Read the model definition and answer for the solid it produces. Units are mm, in the model's axes. A direction names the side the tool comes from. Round coordinates to 2 decimals unless told otherwise and drop trailing zeros. Write each loop counter-clockwise with the first axis right and the second up, starting at its lowest first coordinate (ties: lowest second). Pieces come first, ordered by that corner, then holes. Notation, with made-up numbers: (15, -23.5) -> (71, -23.5) arc R14 cw to (71, -10.5) -> close; hole circle Ø2 at (47.5, 60.25). An arc over 180 degrees is marked (long way). Return JSON: item names as keys, results as strings. Group by question number.
(1) The mould has two halves that part along X. Classify faces 3 (the flat face through (62, 0, -18)), 4 (the cylindrical face through (95.687, 35.49, -2.573)), 5 (the cylindrical face through (92.912, 35.49, -22.825)), 6 (the flat face through (51.37, 34.51, -18.53)): released by +X, released by -X, zero draft, split by the parting line, or undercut.
(2) A cutting plane is placed at B-B on x = 59. Give the vertices of the cut face in (y, z).
(3) For faces 1 (the flat face through (52.606, 34.51, -14.116)), 2 (the flat face through (62, 70, -18)), determine the directions among +Z, -Z, +X, -X, +Y, -Y from which every point of the face is accessible in a straight line to the end or side of a thin tool.
(4) A cutting plane is placed at D-D on z = -31. Give the vertices of the cut face in (x, y).
(5) Straight lines are drawn through the part: line 1 (Z direction, x = 65, y = 29); line 2 (Z direction, x = 28, y = 29.5); line 3 (Z direction, x = 17.5, y = 16.5). For each, find the intervals that lie inside material, in ascending order.
(6) A cutting plane is placed at A-A on z = -10.5. Give the vertices of the cut face in (x, y), then the cut area to 3 significant figures.
(7) Given pin 1 (5 mm diameter, centred on x = 60.5, y = 34, fed in from +Z); pin 2 (12 mm diameter, centred on y = 23.5, z = -28, fed in from +X); pin 3 (4 mm diameter, centred on x = 67, y = 57, fed in from -Z), each flat-ended and moving along its own axis, determine where each tip first touches the part or whether it passes through.
(8) A cutting plane is placed at C-C on y = 14. Give the vertices of the cut face in (x, z), then the cut area to 3 significant figures.
```python
from build123d import *

# Parameters (mm, degrees)
EXTRUDE_2_DEPTH     = 70
CUT_EXTRUDE_1_DEPTH = 129.452325787
FILLET_1_R          = 10
FILLET_2_R          = 3


with BuildPart() as part:
    # 草图5 → 凸台-拉伸2 (new body)
    with BuildSketch(Plane(origin=(0, 0, 0), x_dir=(1, 0, 0), z_dir=(0, 1, 0))):
        Polygon((0, 0), (99.941085936, -3.432104596), (101.313927774, 36.544329779), align=None)
    extrude(amount=EXTRUDE_2_DEPTH)

    # 草图8 → 切除-拉伸1 (cut, through all)
    with BuildSketch(Plane.XZ):
        Polygon((97.48567579, -28.67108094), (96.55900755, -1.686987737), (22.158644136, -4.241991286), align=None)
    extrude(amount=-CUT_EXTRUDE_1_DEPTH, mode=Mode.SUBTRACT)

    # 圆角1
    fillet_1_edges = [part.edges().sort_by_distance(p)[0] for p in [
        (97.48567579, 35, -28.67108094),
    ]]
    fillet(fillet_1_edges, radius=FILLET_1_R)

    # 圆角2
    fillet_2_edges = [part.edges().sort_by_distance(p)[0] for p in [
        (96.55900755, 35, -1.686987737),
    ]]
    fillet(fillet_2_edges, radius=FILLET_2_R)


solid = part.part
```
Checks:
{
 "1": {"face 3": "zero draft", "face 4": "undercut", "face 5": "undercut", "face 6": "released by -X"},
 "2": {"outline": "(0, -21.28) -> (70, -21.28) -> (70, -16.19) -> (0, -16.19) -> close; (0, -2.98) -> (70, -2.98) -> (70, 2.03) -> (0, 2.03) -> close"},
 "3": {"face 1": "+Y, -Y", "face 2": "+Z, -Z, +X, -X, +Y"},
 "4": {"outline": "(85.94, 0) -> (101.12, 0) -> (101.12, 70) -> (85.94, 70) -> close"},
 "5": {"line 1": "z = -23.45 to -18.14, -2.77 to 2.23", "line 2": "z = -10.1 to -6.14, -4.04 to 0.96", "line 3": "z = -6.31 to 0.6"},
 "6": {"outline": "(29.11, 0) -> (41.46, 0) -> (41.46, 70) -> (29.11, 70) -> close; (96.86, 0) -> (100.42, 0) -> (100.42, 70) -> (96.86, 70) -> close", "area": "1,110 mm^2"},
 "7": {"pin 1": "stops at z = 2.16", "pin 2": "stops at x = 101.23", "pin 3": "stops at z = -24.89"},
 "8": {"outline": "(0, 0) -> (101.31, -36.54) -> (99.94, 3.43) -> close; hole (22.16, -4.24) -> (83.92, -24.27) arc R10 ccw to (97, -14.42) -> (96.66, -4.69) arc R3 ccw to (93.56, -1.79) -> close", "area": "1,040 mm^2"}
}
